Geometry check sheet. Reference: the model listing, model coordinates, mm. Face numbers are marked on the shaded views. A direction names the side the tool comes from. Give positions to 0.01 mm unless a question says otherwise; leave off trailing zeros. Write each loop counter-clockwise with the first axis right and the second up, starting at its lowest first coordinate (ties: lowest second). Pieces come first, ordered by that corner, then holes. Notation, with made-up numbers: M -36,-0.75 L 23,-0.75 A31 ccw 23,34.25 Z; hole C 16.5,59 d3. An arc over 180 degrees is marked long. One line per item, written item: value. Start each with the question number.
1. Gauge pin test, flat ends, axial feed: pin 1 (4.5 mm diameter, centred on x = -35, y = 50, fed in from +Z); pin 2 (3 mm diameter, centred on x = -11, y = 10, fed in from -Z); pin 3 (8 mm diameter, centred on x = -47, y = 27.5, fed in from -Z). Record the tip position at first contact, or that the pin passes through.
2. Cross-section at C-C on x = -31. Record the cut outline in (y, z).
3. Cross-section at A-A on x = -10. Record the cut outline in (y, z), then the cut area to 3 significant figures.
4. Cross-section at B-B on y = 55.5. Record the cut outline in (x, z), then the cut area to 3 significant figures.
5. Cross-section at D-D on y = 10. Record the cut outline in (x, z).
6. Scan lines: line 1 (X direction, y = 25.5, z = -4); line 2 (Y direction, x = -31, z = -5.5); line 3 (X direction, y = 3, z = -6). Record each from-to range of solid material in increasing order.
7. Tool access check on the marked faces 1, 2 and 3. Record the directions out of +Z, -Z, +X, -X, +Y, -Y that give a thin tool (end or side, any length) a straight path to the whole face; none if there is none.
from build123d import *

# Parameters (mm, degrees)
EXTRUDE_1_DEPTH     = 60
SKETCH_3_R          = 2.6
CUT_EXTRUDE_1_DEPTH = 10
SKETCH_4_R          = 2.1
CUT_EXTRUDE_2_DEPTH = 10
EXTRUDE_2_DEPTH     = 3
EXTRUDE_3_DEPTH     = 3
EXTRUDE_4_DEPTH     = 20
EXTRUDE_5_DEPTH     = 20
SKETCH_11_W         = 24
SKETCH_11_H         = 4
SKETCH_11_W_2       = 22.185080678
EXTRUDE_6_DEPTH     = 2


with BuildPart() as part:
    # 草图1 → 凸台-拉伸1 (new body)
    with BuildSketch(Plane(origin=(0, 0, 0), x_dir=(1, 0, 0), z_dir=(0, 1, 0))):
        Polygon((0, 0), (-55, 0), (-55, 5), (-6, 54), (0, 54), align=None)
        Polygon((-4.757359313, 51), (-51.5, 4.257359313), (-51.5, 3), (-3, 3), (-3, 51), align=None, mode=Mode.SUBTRACT)
    extrude(amount=EXTRUDE_1_DEPTH)

    # 草图3 → 切除-拉伸1 (cut)
    with BuildSketch(Plane(origin=(0, 0, -3), x_dir=(-1, 0, 0), z_dir=(0, 0, -1))):
        with Locations((11, 10)):
            Circle(SKETCH_3_R)
        with Locations((31, 10)):
            Circle(SKETCH_3_R)
        with Locations((35, 50)):
            Circle(SKETCH_3_R)
        with Locations((10, 50)):
            Circle(SKETCH_3_R)
    extrude(amount=-CUT_EXTRUDE_1_DEPTH, mode=Mode.SUBTRACT)

    # 草图4 → 切除-拉伸2 (cut)
    with BuildSketch(Plane(origin=(-30, 0, -30), x_dir=(-0.7071067811865511, 0, 0.7071067811865439), z_dir=(-0.7071067811865439, 0, -0.7071067811865511))):
        with Locations((12.426406871, 45)):
            Circle(SKETCH_4_R)
        with Locations((-17.573593129, 45)):
            Circle(SKETCH_4_R)
        with Locations(Location((12.426406871, 15, 0), (0, 0, 180))):
            Circle(SKETCH_4_R)
        with Locations(Location((-17.573593129, 15, 0), (0, 0, 180))):
            Circle(SKETCH_4_R)
    extrude(amount=-CUT_EXTRUDE_2_DEPTH, mode=Mode.SUBTRACT)

    # 草图7 → 凸台-拉伸2 (add)
    with BuildSketch(Plane(origin=(0, 20, 0), x_dir=(-1, 0, 0), z_dir=(0, -1, 0))):
        Polygon((3, 52.757359313), (51.5, 4.257359313), (51.5, 3), (3, 3), align=None)
    extrude(amount=-EXTRUDE_2_DEPTH)

    # 草图8 → 凸台-拉伸3 (add)
    with BuildSketch(Plane(origin=(0, 40, 0), x_dir=(1, 0, 0), z_dir=(0, 1, 0))):
        Polygon((-3, 51), (-4.757359313, 51), (-51.5, 4.257359313), (-51.5, 3), (-3, 3), align=None)
    extrude(amount=-EXTRUDE_3_DEPTH)

    # 草图9 → 凸台-拉伸4 (add)
    with BuildSketch(Plane.XZ):
        Polygon((-20.063260388, -3), (-26.098365074, -29.658994238), (-24.008264838, -31.749094475), (-17.5, -3), align=None)
    extrude(amount=-EXTRUDE_4_DEPTH)

    # 草图10 → 凸台-拉伸5 (add)
    with BuildSketch(Plane(origin=(0, 60, 0), x_dir=(1, 0, 0), z_dir=(0, 1, 0))):
        Polygon((-26.098365074, 29.658994238), (-24.008264838, 31.749094475), (-17.5, 3), (-20.063260388, 3), align=None)
    extrude(amount=-EXTRUDE_5_DEPTH)

    # 草图11 → 凸台-拉伸6 (add)
    with BuildSketch(Plane(origin=(-30, 0, -30), x_dir=(-0.7071067811865511, 0, 0.707106781186544), z_dir=(-0.707106781186544, 0, -0.7071067811865511))):
        with Locations((-2.573593129, 45)):
            Rectangle(SKETCH_11_W, SKETCH_11_H)
        with Locations((-2.702962181, 15)):
            Rectangle(SKETCH_11_W_2, SKETCH_11_H)
    extrude(amount=EXTRUDE_6_DEPTH)


solid = part.part
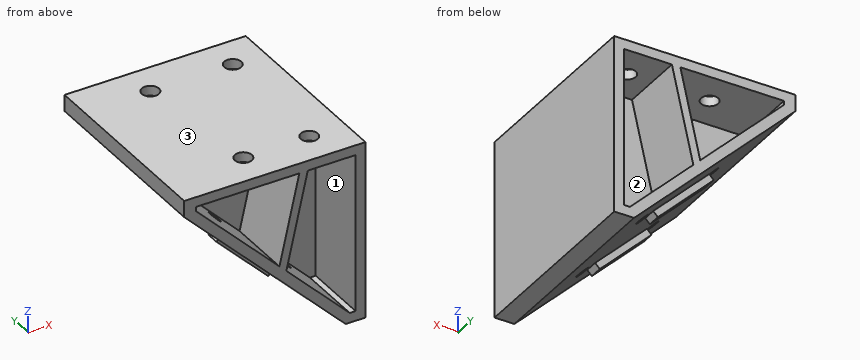
Report:
1. pin 1: stops at z = -18.51
1. pin 2: stops at z = -50.5
1. pin 3: stops at z = -17
2. outline: M 0,-29 L 13,-29 L 13,-31.83 L 17,-31.83 L 17,-29 L 43,-29 L 43,-31.83 L 47,-31.83 L 47,-29 L 60,-29 L 60,-24.76 L 40,-24.76 L 40,-3 L 60,-3 L 60,0 L 12.6,0 L 12.6,-3 L 20,-3 L 20,-24.76 L 0,-24.76 Z; M 0,-3 L 7.4,-3 L 7.4,0 L 0,0 Z; hole M 23,-24.76 L 37,-24.76 L 37,-3 L 23,-3 Z
3. outline: M 0,-50 L 60,-50 L 60,-45.76 L 40,-45.76 L 40,-3 L 47.4,-3 L 47.4,0 L 12.4,0 L 12.4,-3 L 20,-3 L 20,-45.76 L 0,-45.76 Z; M 0,-3 L 7.6,-3 L 7.6,0 L 0,0 Z; M 52.6,-3 L 60,-3 L 60,0 L 52.6,0 Z; hole M 23,-45.76 L 37,-45.76 L 37,-3 L 23,-3 Z
3. area: 661 mm^2
4. outline: M -55,-5 L -6,-54 L 0,-54 L 0,0 L -55,0 Z; hole M -51.5,-4.26 L -26.1,-29.66 L -20.06,-3 L -51.5,-3 Z; hole M -24.01,-31.75 L -4.76,-51 L -3,-51 L -3,-3 L -17.5,-3 Z
4. area: 605 mm^2
5. outline: M -55,-5 L -6,-54 L 0,-54 L 0,0 L -8.4,0 L -8.4,-3 L -3,-3 L -3,-51 L -4.76,-51 L -24.01,-31.75 L -17.5,-3 L -13.6,-3 L -13.6,0 L -28.4,0 L -28.4,-3 L -20.06,-3 L -26.1,-29.66 L -51.5,-4.26 L -51.5,-3 L -33.6,-3 L -33.6,0 L -55,0 Z
6. line 1: x = -55 to -51.5, -3 to 0
6. line 2: y = 20 to 23, 37 to 40
6. line 3: x = -54 to -49.76, -20.74 to -18.18, -3 to 0
7. face 1: -Y
7. face 2: +Y
7. face 3: +Z, +X, -X, +Y, -Y
